```python
from build123d import *

# Parameters (mm, degrees)
F0_R     = 14.2875
F0_R_2   = 12.5
F1_DEPTH = 76.2
F2_W     = 7
F2_H     = 50.8
F3_DEPTH = 14.2885


with BuildPart() as f1:
    # F0 (on Front) → F1 (new body)
    with BuildSketch(Plane.XZ):
        Circle(F0_R)
        Circle(F0_R_2, mode=Mode.SUBTRACT)
    extrude(amount=F1_DEPTH)

    # F2 (on Top) → F3 (cut, through all)
    with BuildSketch(Plane.XY):
        with Locations((0, -38.1)):
            Rectangle(F2_W, F2_H)
    extrude(amount=-F3_DEPTH, mode=Mode.SUBTRACT)


solid = f1.part
```
Here's how the part is built. I have some questions about the finished solid (model axes, mm). A direction names the side the tool comes from. Coordinates: 2 decimals unless noted, no trailing zeros. Loops run counter-clockwise (first coordinate to the right, second up) from the corner with the lowest first, then second, coordinate; pieces in that order, holes last. Notation, with made-up numbers: (-0.5, -30.75) - (15.5, -30.75) arc R30 cw to (15.5, -0.75) - close; hole circle Ø3 at (17.25, -4). An arc over 180 degrees is marked (long way). Return JSON: item names as keys, results as strings. Group by question number.
Item 1: I need wall thicknesses on line 1 (Z direction, x = 0.5, y = -65); line 2 (Z direction, x = -8.5, y = -52.5); line 3 (Z direction, x = 0, y = -53). Which ranges of each line are inside material? Lowest first, please. Write a range as from..to.
Item 2: On a 3-axis mill with a long thin cutter (end or side, diameter ignored), from which of +Z, -Z, +X, -X, +Y, -Y can I reach the whole of each face in a straight line? I mean faces 4 (the face through (-3.5, -38, -13)), 5 (the face through (0, 0, -13)). Say none if no direction works.
Item 3: Will these pins go through, and if not, where does the flat tip stop? P1, Ø2, axis at x = -9, y = -56.5, coming from the -Z side; P2, Ø8, axis at y = -44, z = 10, coming from the -X side; P3, Ø1, axis at x = 10.5, z = -6.5, coming from the +Y side; P4, Ø0.6, axis at y = -48.5, z = -13, coming from the -X side.
Item 4: If we section it at A-A on x = 0: Write out the boundary of the cut face in (y, z).
Item 5: If we section it at D-D on y = -34.5: Write out the boundary of the cut face in (x, z) (1 decimal).
Item 6: If we section it at B-B on z = 0: Write out the boundary of the cut face in (x, y).
Item 7: We'd pull the mould along Y, two halves only. Please class faces 1 (the face through (3.5, -38, -13)), 2 (the face through (0, -76.2, -13)), 3 (the face through (-1.627, -37.567, 12.394)): +Y half, -Y half, draft (parallel to the pull), parting line (faces both ways), or undercut.
Item 8: If we section it at C-C on x = -7.75: Write out the boundary of the cut face in (y, z).
Calculated:
{
 "1": {"line 1": "z = -14.28..-12.49, 12.49..14.28", "line 2": "z = -11.48..-9.17, 9.17..11.48", "line 3": "z = 12.5..14.29"},
 "2": {"face 4": "-Z", "face 5": "+Z, -Z, +X, -X, +Y"},
 "3": {"P1": "stops at z = -11.84", "P2": "stops at x = -12.97", "P3": "stops at y = 0", "P4": "stops at x = -6.55"},
 "4": {"outline": "(-76.2, -14.29) - (-63.5, -14.29) - (-63.5, -12.5) - (-76.2, -12.5) - close; (-76.2, 12.5) - (0, 12.5) - (0, 14.29) - (-76.2, 14.29) - close; (-12.7, -14.29) - (0, -14.29) - (0, -12.5) - (-12.7, -12.5) - close"},
 "5": {"outline": "(-3.5, -13.9) - (-3.5, -12) arc R12.5 cw (long way) to (3.5, -12) - (3.5, -13.9) arc R14.3 ccw (long way) to start"},
 "6": {"outline": "(-14.29, -76.2) - (-12.5, -76.2) - (-12.5, 0) - (-14.29, 0) - close; (12.5, -76.2) - (14.29, -76.2) - (14.29, 0) - (12.5, 0) - close"},
 "7": {"face 1": "undercut", "face 2": "-Y half", "face 3": "draft"},
 "8": {"outline": "(-76.2, -12) - (0, -12) - (0, -9.81) - (-76.2, -9.81) - close; (-76.2, 9.81) - (0, 9.81) - (0, 12) - (-76.2, 12) - close"}
}
